from build123d import *

# Parameters (mm, degrees)
SKETCH1_W            = 3
SKETCH1_H            = 30
BOSS_EXTRUDE1_DEPTH  = 3
SKETCH8_W            = 3
SKETCH8_H            = 3
BOSS_EXTRUDE7_DEPTH  = 20
SKETCH9_W            = 20
SKETCH9_H            = 3
BOSS_EXTRUDE8_DEPTH  = 5
SKETCH12_W           = 3
SKETCH12_H           = 30
BOSS_EXTRUDE10_DEPTH = 3
SKETCH13_W           = 3
SKETCH13_H           = 30
BOSS_EXTRUDE11_DEPTH = 10
FILLET6_R            = 1


with BuildPart() as part:
    # Sketch1 → Boss-Extrude1 (new body)
    with BuildSketch(Plane.XY):
        with Locations((1.5, -15)):
            Rectangle(SKETCH1_W, SKETCH1_H)
    extrude(amount=BOSS_EXTRUDE1_DEPTH)

    # Sketch8 → Boss-Extrude7 (add)
    with BuildSketch(Plane(origin=(0, 0, 0), x_dir=(-1, 0, 0), z_dir=(0, 0, -1))):
        with Locations((-1.5, -28.5)):
            Rectangle(SKETCH8_W, SKETCH8_H)
    extrude(amount=BOSS_EXTRUDE7_DEPTH)

    # Sketch9 → Boss-Extrude8 (add)
    with BuildSketch(Plane.ZY):
        with Locations((-10, -28.5)):
            Rectangle(SKETCH9_W, SKETCH9_H)
    extrude(amount=BOSS_EXTRUDE8_DEPTH)

    # Sketch12 → Boss-Extrude10 (add)
    with BuildSketch(Plane.ZY):
        with Locations((1.5, -15)):
            Rectangle(SKETCH12_W, SKETCH12_H)
    extrude(amount=BOSS_EXTRUDE10_DEPTH)

    # Sketch13 → Boss-Extrude11 (add)
    with BuildSketch(Plane.XY.offset(3)):
        with Locations((-1.5, -15)):
            Rectangle(SKETCH13_W, SKETCH13_H)
    extrude(amount=BOSS_EXTRUDE11_DEPTH)

    # Fillet6
    fillet6_edges = [part.edges().sort_by_distance(p)[0] for p in [
        (-1, -30, -20),
        (-4, -30, 0),
        (-5, -30, -10),
        (-5, -28.5, 0),
        (-3, 0, 6.5),
        (-3, -30, 6.5),
        (1.5, -30, 3),
        (0, -30, 8),
        (-1.5, 0, 13),
        (-3, -15, 13),
        (-1.5, -30, 13),
        (3, -30, -8.5),
    ]]
    fillet(fillet6_edges, radius=FILLET6_R)


solid = part.part
Here's how the part is built. I have some questions about the finished solid (model axes, mm). A direction names the side the tool comes from. Give positions to 0.01 mm unless a question says otherwise; leave off trailing zeros. Order: outer loops, then holes, each group sorted by start corner. A loop starts at its lowest first (then second) coordinate and runs counter-clockwise, first axis right, second up. Notation, with made-up numbers: (44, 68) -> (74, 68) arc R13 cw to (74, 75) -> close; hole circle Ø7 at (-6.75, 84). An arc over 180 degrees is marked (long way). Use a Markdown table: item, result. Add a question column.
Item 1: Imagine slicing it at A-A on y = -20. Please give me the cut outline in (x, z).
Item 2: Imagine slicing it at B-B on x = 1.25. Please give me the cut outline in (y, z).
Item 3: Will these pins go through, and if not, where does the flat tip stop? pin 1 (3 mm diameter, centred on y = -20, z = 10.5, fed in from +X); pin 2 (4 mm diameter, centred on x = -1, y = -4, fed in from -Z); pin 3 (6 mm diameter, centred on y = -19, z = 6, fed in from -X).
Item 4: Imagine slicing it at D-D on x = -2.5. Please give me the cut outline in (y, z).
Item 5: Imagine slicing it at C-C on z = -15. Please give me the cut outline in (x, y), plus the area to 3 significant figures.
Item 6: I need wall thicknesses on line 1 (Y direction, x = -0.75, z = -2.5); line 2 (X direction, y = -8.75, z = 9); line 3 (Z direction, x = 0.5, y = -22.75). Which ranges of each line are inside material? Lowest first, please.
Item 7: For faces 1 (the face through (-0.301, -29.715, 7.577)), 2 (the face through (0, -14, 0)), 3 (the face through (-3.5, -28, 0)), 4 (the face through (0, -15, 8)), 5 (the face through (3, -18, 1)), which set-ups out of +Z, -Z, +X, -X, +Y, -Y let a thin tool reach every point of the face, with its end or its side?
Data:
| question | item | result |
|---|---|---|
| 1 | outline | (-3, 0) -> (3, 0) -> (3, 3) -> (0, 3) -> (0, 13) -> (-2, 13) arc R1 ccw to (-3, 12) -> close |
| 2 | outline | (-30, -19) arc R1 ccw to (-29, -20) -> (-27, -20) -> (-27, 0) -> (0, 0) -> (0, 3) -> (-29, 3) arc R1 ccw to (-30, 2) -> close |
| 3 | pin 1 | stops at x = 0 |
| 3 | pin 2 | stops at z = 0 |
| 3 | pin 3 | stops at x = -3 |
| 4 | outline | (-30, -19) arc R1 ccw to (-29, -20) -> (-27, -20) -> (-27, 0) -> (-0.13, 0) -> (-0.13, 12) arc R0.87 ccw to (-1, 12.87) -> (-29, 12.87) arc R0.87 ccw to (-29.87, 12) -> (-29.87, -0.5) arc R1 ccw to (-30, -1) -> close |
| 5 | outline | (-5, -29) arc R1 ccw to (-4, -30) -> (2, -30) arc R1 ccw to (3, -29) -> (3, -27) -> (-5, -27) -> close |
| 5 | area | 23.6 mm² |
| 6 | line 1 | y = -30 to -27 |
| 6 | line 2 | x = -3 to 0 |
| 6 | line 3 | z = 0 to 3 |
| 7 | face 1 | +Z, +X, -Y |
| 7 | face 2 | -Z, +X, -X, +Y |
| 7 | face 3 | +Z, -X, +Y, -Y |
| 7 | face 4 | +Z, +X, +Y, -Y |
| 7 | face 5 | +Z, -Z, +X, +Y, -Y |
